For this review, use the dimensioned drawing (mm, ordinates from the lowest corner) and the shaded views. Round coordinates to 2 decimals unless told otherwise and drop trailing zeros. Order: outer loops, then holes, each group sorted by start corner. A loop starts at its lowest first (then second) coordinate and runs counter-clockwise, first axis right, second up. Notation, with made-up numbers: M -33.75,46 L 20.25,46 A27 cw 20.25,71 Z; hole C 52,33 d3. An arc over 180 degrees is marked long. Use a Markdown table: item, result. Add a question column.
1. Consider section A-A on y = 123.5. State the section outline as (x, z) points.
2. Insertion check: P1, Ø1, axis at y = 55, z = 2, coming from the -X side. The pin has a flat end and moves straight along its axis. Give the tip position at first contact, or say it passes through.
3. Consider section B-B on x = 116. State the section outline as (y, z) points, then the cut area to 3 significant figures.
4. Consider section C-C on x = 223.5. State the section outline as (y, z) points.
5. To check wall thickness, follow probe 1 along Y at (x, z) = (116, 0.95); probe 2 along X at (y, z) = (8.5, 1.8); probe 3 along X at (y, z) = (116.5, 1.25). State the ranges of each line that lie inside material, in increasing order.
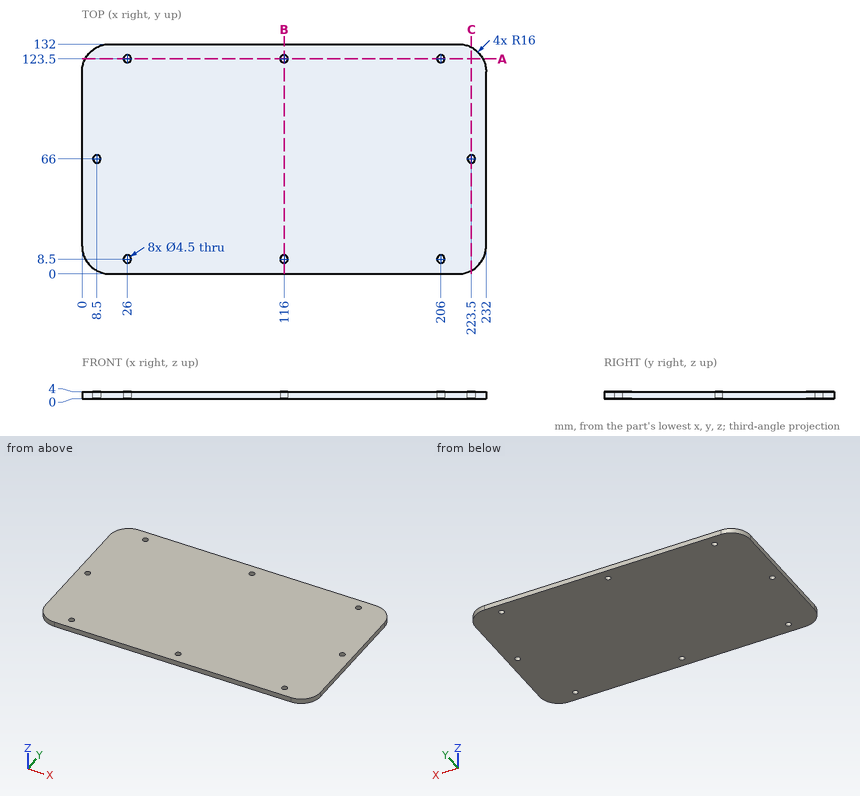
Answer block:
| question | item | result |
|---|---|---|
| 1 | outline | M 1.87,0 L 23.75,0 L 23.75,4 L 1.87,4 Z; M 28.25,0 L 113.75,0 L 113.75,4 L 28.25,4 Z; M 118.25,0 L 203.75,0 L 203.75,4 L 118.25,4 Z; M 208.25,0 L 230.13,0 L 230.13,4 L 208.25,4 Z |
| 2 | P1 | x = 0 |
| 3 | outline | M 0,0 L 6.25,0 L 6.25,4 L 0,4 Z; M 10.75,0 L 121.25,0 L 121.25,4 L 10.75,4 Z; M 125.75,0 L 132,0 L 132,4 L 125.75,4 Z |
| 3 | area | 492 mm^2 |
| 4 | outline | M 1.87,0 L 63.75,0 L 63.75,4 L 1.87,4 Z; M 68.25,0 L 130.13,0 L 130.13,4 L 68.25,4 Z |
| 5 | probe 1 | 0 to 6.25, 10.75 to 121.25, 125.75 to 132 |
| 5 | probe 2 | 1.87 to 23.75, 28.25 to 113.75, 118.25 to 203.75, 208.25 to 230.13 |
| 5 | probe 3 | 0.01 to 231.99 |
